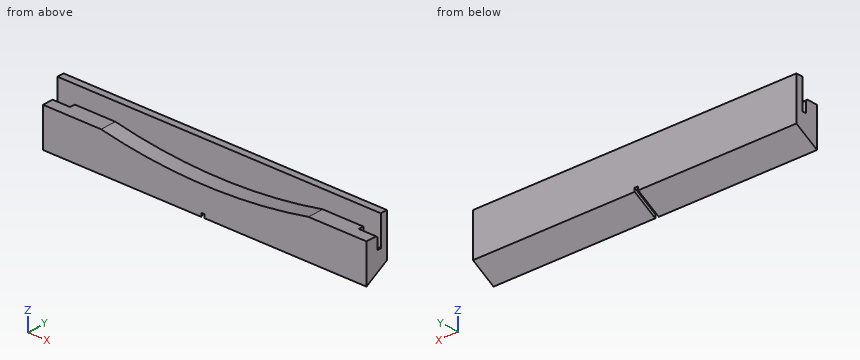
```python
from build123d import *

# Parameters (mm, degrees)
SKETCH_2_W                  = 93.1
SKETCH_2_H                  = 10
EXTRUDE_1_DEPTH             = 3.5
SKETCH_4_W                  = 93.1
SKETCH_4_H                  = 6.5
EXTRUDE_2_DEPTH             = 1.1
SKETCH_5_W                  = 93.1
SKETCH_5_H                  = 10
EXTRUDE_3_DEPTH             = 2
CUT_EXTRUDE_1_DEPTH         = 94.867832616
SKETCH_7_W                  = 83.1
SKETCH_7_H                  = 1.1
EXTRUDE_4_DEPTH             = 3.5
CHAMFER_1_SIZE              = 0.4
CUT_EXTRUDE_2_REACH         = 95.868
SKETCH_8_R                  = 150
SKETCH_9_W                  = 93.1
SKETCH_9_H                  = 2
EXTRUDE_5_DEPTH             = 5
EXTRUDE_5_DIRECTION_2_REACH = 95.868
SKETCH_10_W                 = 93.1
SKETCH_10_H                 = 7.621023553
EXTRUDE_6_DEPTH             = 1
SKETCH_11_W                 = 1
SKETCH_11_H                 = 7.621023553
CUT_EXTRUDE_3_DEPTH         = 1


with BuildPart() as part:
    # 草图2 → 凸台-拉伸1 (new body)
    with BuildSketch(Plane(origin=(0, 0, 0), x_dir=(1, 0, 0), z_dir=(0, 1, 0))):
        with Locations((46.55, 5)):
            Rectangle(SKETCH_2_W, SKETCH_2_H)
    extrude(amount=EXTRUDE_1_DEPTH)

    # 草图4 → 凸台-拉伸2 (add)
    with BuildSketch(Plane(origin=(0, 3.5, 0), x_dir=(1, 0, 0), z_dir=(0, 1, 0))):
        with Locations((46.55, 6.75)):
            Rectangle(SKETCH_4_W, SKETCH_4_H)
    extrude(amount=EXTRUDE_2_DEPTH)

    # 草图5 → 凸台-拉伸3 (add)
    with BuildSketch(Plane(origin=(0, 4.6, 0), x_dir=(1, 0, 0), z_dir=(0, 1, 0))):
        with Locations((46.55, 5)):
            Rectangle(SKETCH_5_W, SKETCH_5_H)
    extrude(amount=EXTRUDE_3_DEPTH)

    # 草图6 → 切除-拉伸1 (cut, through all)
    with BuildSketch(Plane.ZY):
        Polygon((-10, 0), (-6.189488223, 6.6), (-10, 6.6), align=None)
    extrude(amount=-CUT_EXTRUDE_1_DEPTH, mode=Mode.SUBTRACT)

    # 草图7 → 凸台-拉伸4 (add)
    with BuildSketch(Plane.XY.offset(-3.5)):
        with Locations((46.55, 4.05)):
            Rectangle(SKETCH_7_W, SKETCH_7_H)
    extrude(amount=EXTRUDE_4_DEPTH)

    # 倒角1
    chamfer_1_edges = [part.edges().sort_by_distance(p)[0] for p in [
        (90.6, 3.5, 0),
        (2.5, 3.5, 0),
    ]]
    chamfer(chamfer_1_edges, length=CHAMFER_1_SIZE)

    # 草图8 → 切除-拉伸2 (cut, up to next)
    with BuildSketch(Plane.XZ, mode=Mode.PRIVATE) as cut_extrude_2_sk1:
        with Locations((46.55, 147)):
            Circle(SKETCH_8_R)
    cut_extrude_2_tool1 = extrude(cut_extrude_2_sk1.sketch, amount=-CUT_EXTRUDE_2_REACH, mode=Mode.PRIVATE) & part.part
    add(cut_extrude_2_tool1.solids().sort_by_distance((46.55, 0, 147))[0], mode=Mode.SUBTRACT)

    # 草图9 → 凸台-拉伸5 (add)
    with BuildSketch(Plane.XY):
        with Locations((46.55, 5.6)):
            Rectangle(SKETCH_9_W, SKETCH_9_H)
    extrude(amount=EXTRUDE_5_DEPTH)

    # 草图9 → 凸台-拉伸5 direction 2 (add, up to next)
    with BuildSketch(Plane.XY, mode=Mode.PRIVATE) as extrude_5_direction_2_sk1:
        with Locations((46.55, 5.6)):
            Rectangle(SKETCH_9_W, SKETCH_9_H)
    extrude_5_direction_2_tool1 = extrude(extrude_5_direction_2_sk1.sketch, amount=-EXTRUDE_5_DIRECTION_2_REACH, mode=Mode.PRIVATE) - part.part
    add(extrude_5_direction_2_tool1.solids().sort_by_distance((46.55, 5.6, 0))[0])

    # 草图10 → 凸台-拉伸6 (add, along a direction that is not the sketch's normal)
    with BuildSketch(Plane(origin=(0, 4.330127019, -7.5), x_dir=(-1, 0, 0), z_dir=(0, 0.4999999999999947, -0.8660254037844417))):
        with Locations((-46.55, -1.189488223)):
            Rectangle(SKETCH_10_W, SKETCH_10_H)
    extrude(amount=EXTRUDE_6_DEPTH, dir=(0, 0, -1))

    # 草图11 → 切除-拉伸3 (cut, along a direction that is not the sketch's normal)
    with BuildSketch(Plane(origin=(0, 4.763139721, -8.25), x_dir=(-1, 0, 0), z_dir=(0, 0.49999999999999484, -0.8660254037844418))):
        with Locations((-46.05, -1.689488223)):
            Rectangle(SKETCH_11_W, SKETCH_11_H)
    extrude(amount=-CUT_EXTRUDE_3_DEPTH, dir=(0, 0, -1), mode=Mode.SUBTRACT)


solid = part.part
```
Build history of the part. All positions in model axes, mm. Give positions to 0.01 mm unless a question says otherwise; leave off trailing zeros. Loops run counter-clockwise (first coordinate to the right, second up) from the corner with the lowest first, then second, coordinate; pieces in that order, holes last.
1) Band-saw the part on B-B on x = 11. List the corners of the cut face in (y, z).
Values follow:
outline: (0, -11) - (6.6, -7.19) - (6.6, 5) - (4.6, 5) - (4.6, 0) - (0, 0) - close
2) Probe line 1 along Z through (x, y) = (88, 1.75); line 2 along Y through (x, z) = (31, 4); line 3 along Z through (x, y) = (13.5, 1.25). List the from-to ranges inside material, lowest first.
Values follow:
line 1: z = -9.99 to 0
line 2: y = 4.6 to 6.6
line 3: z = -10.28 to 0
3) Band-saw the part on D-D on y = 1.75. List the corners of the cut face in (x, z).
Values follow:
outline: (0, -9.99) - (45.55, -9.99) - (45.55, -8.99) - (46.55, -8.99) - (46.55, -9.99) - (93.1, -9.99) - (93.1, 0) - (76.4, 0) arc R150 cw to (16.7, 0) - (0, 0) - close
4) Band-saw the part on A-A on y = 5.5. List the corners of the cut face in (x, z), then the cut area to 3 significant figures.
Values follow:
outline: (0, -7.82) - (45.55, -7.82) - (45.55, -6.82) - (46.55, -6.82) - (46.55, -7.82) - (93.1, -7.82) - (93.1, 5) - (0, 5) - close
area: 1,190 mm2
5) Drop a flat-ended pin along its axis: P1, Ø9.5, axis at x = 59, z = 3, coming from the -Y side. Give the stop position or say it passes through.
Values follow:
P1: stops at y = 4.6
6) Band-saw the part on C-C on z = -8.5. List the corners of the cut face in (x, y).
Values follow:
outline: (0, 0) - (93.1, 0) - (93.1, 4.33) - (46.55, 4.33) - (46.55, 2.6) - (45.55, 2.6) - (45.55, 4.33) - (0, 4.33) - close
